Part model, mm, in its own coordinate system. A direction names the side the tool comes from. Round coordinates to 2 decimals unless told otherwise and drop trailing zeros. Loops run counter-clockwise (first coordinate to the right, second up) from the corner with the lowest first, then second, coordinate; pieces in that order, holes last. Notation, with made-up numbers: (19, 78.5) -> (44, 78.5) arc R21 cw to (44, 97.5) -> close; hole circle Ø7 at (68.25, 18). An arc over 180 degrees is marked (long way). Answer as CSV lines item,"result".
from build123d import *

# Parameters (mm, degrees)
F0_W     = 609.6
F0_H     = 520.7
F0_R     = 25.4
F0_R_2   = 15.875
F1_DEPTH = 1.58242
F2_W     = 571.5
F2_H     = 492.125
F2_R     = 25.4
F2_R_2   = 15.875
F3_DEPTH = 0.79375
F4_W     = 571.5
F4_H     = 422.275
F4_R     = 25.4
F4_R_2   = 15.875
F5_DEPTH = 3.175
F6_W     = 225.425
F6_H     = 304.8
F6_R     = 25.4
F6_R_2   = 15.875
F7_DEPTH = 127


with BuildPart() as f1:
    # F0 (on Top) → F1 (new body)
    with BuildSketch(Plane.XY):
        with Locations((304.8, 260.35)):
            Rectangle(F0_W, F0_H)
        with Locations((508, 266.7)):
            Circle(F0_R, mode=Mode.SUBTRACT)
        with Locations((403.225, 412.75)):
            Circle(F0_R_2, mode=Mode.SUBTRACT)
        with Locations((555.625, 412.75)):
            Circle(F0_R_2, mode=Mode.SUBTRACT)
    extrude(amount=F1_DEPTH)

    # F2 (on face) → F3 (join)
    with BuildSketch(Plane.XY.offset(1.58242)):
        with Locations((304.8, 265.1125)):
            Rectangle(F2_W, F2_H)
        with Locations((508, 266.7)):
            Circle(F2_R, mode=Mode.SUBTRACT)
        with Locations((403.225, 412.75)):
            Circle(F2_R_2, mode=Mode.SUBTRACT)
        with Locations((555.625, 412.75)):
            Circle(F2_R_2, mode=Mode.SUBTRACT)
    extrude(amount=F3_DEPTH)

    # F4 (on face) → F5 (join)
    with BuildSketch(Plane.XY.offset(2.37617)):
        with Locations((304.8, 300.0375)):
            Rectangle(F4_W, F4_H)
        with Locations((508, 266.7)):
            Circle(F4_R, mode=Mode.SUBTRACT)
        with Locations((403.225, 412.75)):
            Circle(F4_R_2, mode=Mode.SUBTRACT)
        with Locations((555.625, 412.75)):
            Circle(F4_R_2, mode=Mode.SUBTRACT)
    extrude(amount=F5_DEPTH)

    # F6 (on face) → F7 (join)
    with BuildSketch(Plane.XY.offset(2.37617)):
        with Locations((477.8375, 336.55)):
            Rectangle(F6_W, F6_H)
        with Locations((508, 266.7)):
            Circle(F6_R, mode=Mode.SUBTRACT)
        with Locations((403.225, 412.75)):
            Circle(F6_R_2, mode=Mode.SUBTRACT)
        with Locations((555.625, 412.75)):
            Circle(F6_R_2, mode=Mode.SUBTRACT)
    extrude(amount=F7_DEPTH)


solid = f1.part
Q1. Two-plate mould, pull along Y, no slides. Class faces 1 (the face through (476, 184.15, 67)), 2 (the face through (237, 303, 5.551)), 3 (the face through (553.56, 428.49, 63.78)), 4 (the face through (476, 488.95, 67)): pulls with the +Y half, pulls with the -Y half, needs draft (parallel to the pull), parting line crosses it, or undercut.
Geometry results:
face 1,"pulls with the -Y half"
face 2,"needs draft"
face 3,"undercut"
face 4,"pulls with the +Y half"
Q2. Saw through at A-A, the plane y = 266.7. Write the cut outline in (x, z) (3 decimals).
Geometry results:
outline,"(0, 0) -> (482.6, 0) -> (482.6, 129.376) -> (365.125, 129.376) -> (365.125, 5.551) -> (19.05, 5.551) -> (19.05, 1.582) -> (0, 1.582) -> close; (533.4, 0) -> (609.6, 0) -> (609.6, 1.582) -> (590.55, 1.582) -> (590.55, 129.376) -> (533.4, 129.376) -> close"
Q3. Saw through at C-C, the plane z = 13.5. Write the cut outline in (x, y) (3 decimals).
Geometry results:
outline,"(365.125, 184.15) -> (590.55, 184.15) -> (590.55, 488.95) -> (365.125, 488.95) -> close; hole circle Ø31.75 at (403.225, 412.75); hole circle Ø50.8 at (508, 266.7); hole circle Ø31.75 at (555.625, 412.75)"
Q4. Saw through at B-B, the plane x = 508. Write the cut outline in (y, z) (3 decimals).
Geometry results:
outline,"(0, 0) -> (241.3, 0) -> (241.3, 129.376) -> (184.15, 129.376) -> (184.15, 5.551) -> (88.9, 5.551) -> (88.9, 2.376) -> (19.05, 2.376) -> (19.05, 1.582) -> (0, 1.582) -> close; (292.1, 0) -> (520.7, 0) -> (520.7, 1.582) -> (511.175, 1.582) -> (511.175, 5.551) -> (488.95, 5.551) -> (488.95, 129.376) -> (292.1, 129.376) -> close"
Q5. Saw through at D-D, the plane y = 158. Write the cut outline in (x, z).
Geometry results:
outline,"(0, 0) -> (609.6, 0) -> (609.6, 1.58) -> (590.55, 1.58) -> (590.55, 5.55) -> (19.05, 5.55) -> (19.05, 1.58) -> (0, 1.58) -> close"
Q6. Which spindle directions (+Z, -Z, +X, -X, +Y, -Y) get a long thin tool onto all of the face, cutting with end or side? Do faces 5 (the face through (590.55, 316, 65)), 6 (the face through (301, 264, 0)), 7 (the face through (301, 54, 2.376)), 8 (the face through (401.16, 428.49, 63.78)), 9 (the face through (365.125, 334, 67)). Say none if no direction does.
Geometry results:
face 5,"+Z, +X, +Y, -Y"
face 6,"-Z, +X, -X, +Y, -Y"
face 7,"+Z, +X, -X, -Y"
face 8,"+Z, -Z"
face 9,"+Z, -X, +Y, -Y"
Q7. Drop flat-ended pins along their axis: P1, Ø3, axis at x = 304, y = 366, coming from the +Z side; P2, Ø21, axis at x = 368.5, y = 53, coming from the +Z side; P3, Ø5, axis at y = 392.5, z = 64, coming from the +X side. Give the stop position or say it passes through.
Geometry results:
P1,"z = 5.55"
P2,"z = 2.38"
P3,"x = 590.55"
Q8. Drill centre lines: line 1 along X through (y, z) = (266, 53) (3 decimals); line 2 along Y through (x, z) = (508, 100.5); line 3 along Z through (x, y) = (257.5, 240). Where is each one in solid material? Low to high.
Geometry results:
line 1,"365.125 to 482.61, 533.39 to 590.55"
line 2,"184.15 to 241.3, 292.1 to 488.95"
line 3,"0 to 5.55"
